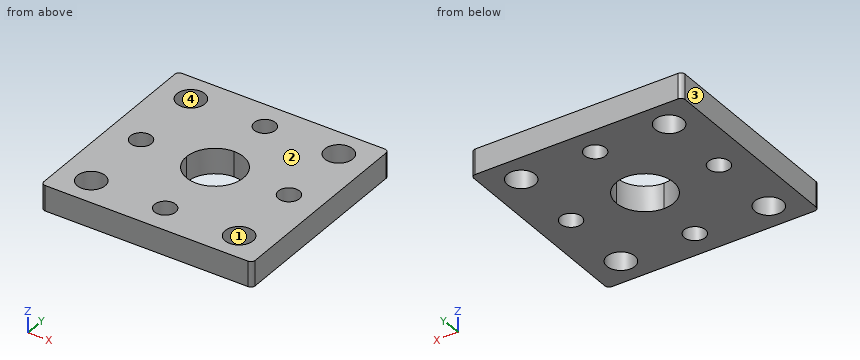
```python
from build123d import *

# Parameters (mm, degrees)
SKETCH_1_W          = 50
SKETCH_1_H          = 48
EXTRUDE_1_DEPTH     = 6
FILLET_1_R          = 1
SKETCH_2_R          = 3.3
CUT_EXTRUDE_1_DEPTH = 70.570108524
HOLE_WIZARD_M6_2_D  = 5


with BuildPart() as part:
    # 草图1 → 凸台-拉伸1 (new body)
    with BuildSketch(Plane.XY):
        with Locations((25, -24)):
            Rectangle(SKETCH_1_W, SKETCH_1_H)
    extrude(amount=EXTRUDE_1_DEPTH)

    # 圆角1
    fillet_1_edges = [part.edges().sort_by_distance(p)[0] for p in [
        (0, 0, 3),
        (50, 0, 3),
        (50, -48, 3),
        (0, -48, 3),
    ]]
    fillet(fillet_1_edges, radius=FILLET_1_R)

    # 草图2 → 切除-拉伸1 (cut, through all)
    with BuildSketch(Plane.XY.offset(6)):
        with Locations((7.5, -6.5)):
            Circle(SKETCH_2_R)
        with Locations((42.5, -6.5)):
            Circle(SKETCH_2_R)
        with Locations((42.5, -41.5)):
            Circle(SKETCH_2_R)
        with Locations((7.5, -41.5)):
            Circle(SKETCH_2_R)
        with BuildLine():
            Line((25, -24), (31.75, -24))
            ThreePointArc((31.75, -24), (29.772970773, -19.227029227), (25, -17.25))
            Line((25, -17.25), (25, -24))
        make_face()
        with BuildLine():
            Line((18.25, -24), (25, -24))
            Line((25, -24), (25, -17.25))
            ThreePointArc((25, -17.25), (20.227029227, -19.227029227), (18.25, -24))
        make_face()
        with BuildLine():
            ThreePointArc((25, -30.75), (29.772970773, -28.772970773), (31.75, -24))
            Line((31.75, -24), (25, -24))
            Line((25, -24), (25, -30.75))
        make_face()
        with BuildLine():
            Line((25, -30.75), (25, -24))
            Line((25, -24), (18.25, -24))
            ThreePointArc((18.25, -24), (20.227029227, -28.772970773), (25, -30.75))
        make_face()
    extrude(amount=-CUT_EXTRUDE_1_DEPTH, mode=Mode.SUBTRACT)

    # M6 螺纹孔2 (through all)
    with Locations(Plane.XY.offset(6)):
        with Locations((25, -6.5), (42.5, -24), (25, -41.5), (7.5, -24)):
            Hole(HOLE_WIZARD_M6_2_D / 2)


solid = part.part
```
The listing builds one solid part. Answer for the finished solid, in the listing's coordinates (mm). Face numbers are marked on the shaded views. Round coordinates to 2 decimals unless told otherwise and drop trailing zeros. Order: outer loops, then holes, each group sorted by start corner. A loop starts at its lowest first (then second) coordinate and runs counter-clockwise, first axis right, second up. Notation, with made-up numbers: (18, 77.5) - (63, 77.5) arc R11 cw to (63, 82.5) - close; hole circle Ø10 at (60, 4). An arc over 180 degrees is marked (long way). Put each result on its own line as item: value. Start each with the question number.
(1) Find section B-B (z = 1.35). State how many separate pieces and enclosed holes the cut face has, plus the area to 3 significant figures.
(2) Straight lines are drawn through the part: probe 1 along Y at (x, z) = (7.5, 1.55); probe 2 along Y at (x, z) = (6, 5.2); probe 3 along X at (y, z) = (-24.5, 3.05). For each, find the intervals that lie inside material, in ascending order. Write a range as from..to.
(3) Find section A-A (y = -6.5). Give the vertices of the cut face in (x, z).
(4) Given P1, Ø8, axis at x = 42.5, y = -24, coming from the +Z side; P2, Ø4, axis at x = 25, y = -41.5, coming from the +Z side, each flat-ended and moving along its own axis, determine where each tip first touches the part or whether it passes through.
(5) Find section D-D (x = 28.5). Give the vertices of the cut face in (y, z).
(6) Find section C-C (x = 7.5). Give the vertices of the cut face in (y, z), plus the area to 3 significant figures.
(7) Determine the mould class of the marked faces 1, 2, 3 and 4 for opening direction X: released by +X, released by -X, zero draft, split by the parting line, or undercut.
Reply:
1. separate pieces: 1
1. enclosed holes: 9
1. area: 2,040 mm^2
2. probe 1: -48..-44.8, -38.2..-26.5, -21.5..-9.8, -3.2..0
2. probe 2: -48..-44.44, -38.56..-26, -22..-9.44, -3.56..0
2. probe 3: 0..5.05, 9.95..18.27, 31.73..40.05, 44.95..50
3. outline: (0, 0) - (4.2, 0) - (4.2, 6) - (0, 6) - close; (10.8, 0) - (22.5, 0) - (22.5, 6) - (10.8, 6) - close; (27.5, 0) - (39.2, 0) - (39.2, 6) - (27.5, 6) - close; (45.8, 0) - (50, 0) - (50, 6) - (45.8, 6) - close
4. P1: z = 6
4. P2: through
5. outline: (-48, 0) - (-29.77, 0) - (-29.77, 6) - (-48, 6) - close; (-18.23, 0) - (0, 0) - (0, 6) - (-18.23, 6) - close
6. outline: (-48, 0) - (-44.8, 0) - (-44.8, 6) - (-48, 6) - close; (-38.2, 0) - (-26.5, 0) - (-26.5, 6) - (-38.2, 6) - close; (-21.5, 0) - (-9.8, 0) - (-9.8, 6) - (-21.5, 6) - close; (-3.2, 0) - (0, 0) - (0, 6) - (-3.2, 6) - close
6. area: 179 mm^2
7. face 1: undercut
7. face 2: zero draft
7. face 3: released by -X
7. face 4: undercut
